Model file for the job. Use its own axes, mm. Face numbers are marked on the shaded views. A direction names the side the tool comes from. Coordinates: 2 decimals unless noted, no trailing zeros. Write each loop counter-clockwise with the first axis right and the second up, starting at its lowest first coordinate (ties: lowest second). Pieces come first, ordered by that corner, then holes. Notation, with made-up numbers: (50.25, -2) -> (108.25, -2) arc R18 cw to (108.25, 27) -> close; hole circle Ø1 at (40, 70). An arc over 180 degrees is marked (long way). Write item = value, one per line. Start each with the question number.
from build123d import *

# Parameters (mm, degrees)
F1_DEPTH    = 40
F2_R        = 7.5
F3_R        = 2
F4_W        = 38.5823002379
F4_H        = 36
F5_DEPTH    = 25.4
F6_R        = 5
F7_T1_DEPTH = 16.8444406885
F7_T3_DEPTH = 16.8444406885


# Not quite as in the source:
# - a fillet or chamfer that OpenCascade refuses, or shapes differently, is made with other operations: its cross-section is extruded or revolved along the edge and cut away or added


with BuildPart() as f1:
    # F0 (on Front) → F1 (new body)
    with BuildSketch(Plane.XZ):
        with BuildLine():
            ThreePointArc((-19.4176997621, 10), (-39.3462840799, 7.4593677642), (-58, 0))
            Line((-58, 0), (-19.4176997621, 0))
            Line((-19.4176997621, 0), (-19.4176997621, 10))
        make_face()
        Polygon((0, 5), (0, 0), (-10, 0), (-11.9571349147, 5), (-13.9571349147, 5), (-12, 0), (-13.5034299327, 0), (-17.4176997621, 10), (-19.4176997621, 10), (-19.4176997621, 0), (-58, 0), (-58, -2), (2, -2), (2, 5), align=None)
    extrude(amount=-F1_DEPTH)

    # F2
    f2_edges = [f1.edges().sort_by_distance(p)[0] for p in [
        (-10, 20, 0),
    ]]
    fillet(f2_edges, radius=F2_R)

    # F3
    f3_edges = [f1.edges().sort_by_distance(p)[0] for p in [
        (0, 20, 0),
    ]]
    fillet(f3_edges, radius=F3_R)

    # F4 (on face) → F5 (cut)
    with BuildSketch(Plane.XY.offset(10)):
        with Locations((-38.7088498811, 20)):
            Rectangle(F4_W, F4_H)
    extrude(amount=-F5_DEPTH, mode=Mode.SUBTRACT)

    # F6
    f6_edges = [f1.edges().sort_by_distance(p)[0] for p in [
        (-19.4177, 2, 4),
        (-19.4177, 38, 4),
    ]]
    fillet(f6_edges, radius=F6_R)

    # F7: fillet of radius 5 on 2 edges, made by hand

    # F7_s2 → F7_t1 (cut)
    with BuildSketch(Plane.XZ.offset(-9.4222203443)):
        with BuildLine():
            ThreePointArc((-58, -2), (-57.0714339554, -0.0080127697), (-55.3783893775, 1.3933608716))
            ThreePointArc((-55.3783893775, 1.3933608716), (-56.6957053109, 0.7089301814), (-58, 0))
            Line((-58, 0), (-58, -2))
        make_face()
    extrude(amount=F7_T1_DEPTH, mode=Mode.SUBTRACT)

    # F7_s4 → F7_t3 (cut)
    with BuildSketch(Plane.XZ.offset(-47.4222203443)):
        with BuildLine():
            ThreePointArc((-58, -2), (-57.0714339554, -0.0080127697), (-55.3783893775, 1.3933608716))
            ThreePointArc((-55.3783893775, 1.3933608716), (-56.6957053109, 0.7089301814), (-58, 0))
            Line((-58, 0), (-58, -2))
        make_face()
    extrude(amount=F7_T3_DEPTH, mode=Mode.SUBTRACT)


solid = f1.part
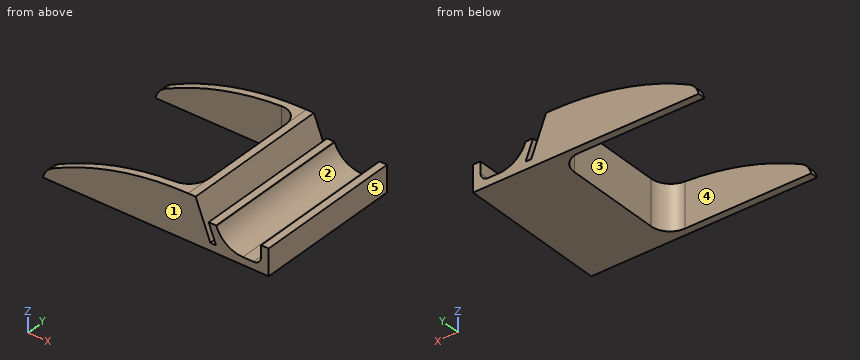
(1) Saw through at C-C (z = 3). Give the cut face in (x, y).
(2) Saw through at D-D (x = -46). Give the cut face in (y, z), then the cut area to 3 significant figures.
(3) 3-axis set-ups, long thin cutter, end or side, ignore diameter. For the marked faces 4 and 5: which of +Z, -Z, +X, -X, +Y, -Y reach the whole face in a straight line?
(4) Drop flat-ended pins along their axis: pin 1 Ø4 at (y, z) = (9, 0.5) entering from -X; pin 2 Ø5 at (y, z) = (5, 1) entering from -X; pin 3 Ø1.6 at (x, y) = (-13.5, 21.5) entering from +Z. Give the stop position or say it passes through.
(5) Drill centre lines: line 1 along X through (y, z) = (21, 1.75) (3 decimals); line 2 along Y through (x, z) = (-25, 1.75); line 3 along X through (y, z) = (8, 4.5). Where is each one in solid material? Low to high.
(6) Mould opens along Y. For the marked faces 1, 2 and 3 say: released by +Y, released by -Y, zero draft, split by the parting line, or undercut.
(7) Saw through at B-B (x = -32.5). Give the cut face in (y, z).
(8) Saw through at A-A (y = 11.5). Give the cut face in (x, z).
Returned:
q1.outline = (-52.02, 0) -> (-14.68, 0) -> (-14.68, 40) -> (-52.02, 40) -> (-52.02, 38) -> (-24.42, 38) arc R5 cw to (-19.42, 33) -> (-19.42, 7) arc R5 cw to (-24.42, 2) -> (-52.02, 2) -> close; (-13.17, 0) -> (-10.88, 0) -> (-10.88, 40) -> (-13.17, 40) -> close; (0, 0) -> (2, 0) -> (2, 40) -> (0, 40) -> close
q2.outline = (0, -2) -> (2, -2) -> (2, 5.42) -> (0, 5.42) -> close; (38, -2) -> (40, -2) -> (40, 5.42) -> (38, 5.42) -> close
q2.area = 29.7 mm2
q3.face_4 = +Z, -Z, -X
q3.face_5 = +Z, -Z, +X, +Y, -Y
q4.pin_1 = -19.42
q4.pin_2 = -22.24
q4.pin_3 = 5
q5.line_1 = -19.418 to -14.188, -12.685 to -9.697, -0.016 to 2
q5.line_2 = 0 to 2, 38 to 40
q5.line_3 = -19.42 to -15.26, -13.76 to -11.76, 0 to 2
q6.face_1 = released by -Y
q6.face_2 = zero draft
q6.face_3 = undercut
q7.outline = (0, -2) -> (2, -2) -> (2, 8.92) -> (0, 8.92) -> close; (38, -2) -> (40, -2) -> (40, 8.92) -> (38, 8.92) -> close
q8.outline = (-19.42, -2) -> (2, -2) -> (2, 5) -> (0, 5) -> (0, 2) arc R2 cw to (-2, 0) -> (-4.88, 0) arc R7.5 cw to (-11.87, 4.77) -> (-11.96, 5) -> (-13.96, 5) -> (-12, 0) -> (-13.5, 0) -> (-17.42, 10) -> (-19.42, 10) -> close
